Source: CAD feature listing. Evaluate the final solid. Frame: model axes, mm. A direction names the side the tool comes from. Round coordinates to 2 decimals unless told otherwise and drop trailing zeros. Loops run counter-clockwise (first coordinate to the right, second up) from the corner with the lowest first, then second, coordinate; pieces in that order, holes last. Notation, with made-up numbers: (-39, -26.75) - (-26, -26.75) arc R23 ccw to (-26, -5.75) - close; hole circle Ø8 at (85, 48.5). An arc over 180 degrees is marked (long way). Use CSV: the item, a comma, the result in double quotes. Start each with the question number.
from build123d import *

# Parameters (mm, degrees)
F0_W     = 250
F0_H     = 300
F1_DEPTH = 300
F2_W     = 250
F2_H     = 250
F3_DEPTH = 250.001


with BuildPart() as f1:
    # F0 (on Front) → F1 (new body)
    with BuildSketch(Plane.XZ):
        with Locations((-125, 150)):
            Rectangle(F0_W, F0_H)
    extrude(amount=F1_DEPTH)

    # F2 (on face) → F3 (cut, through all)
    with BuildSketch(Plane.YZ):
        with Locations((-150, 150)):
            Rectangle(F2_W, F2_H)
    extrude(amount=-F3_DEPTH, mode=Mode.SUBTRACT)


solid = f1.part
1. Mould query, pull axis Z, two halves, no side actions, for faces 1 (the flat face through (-123, -275, 148)), 2 (the flat face through (-127, -148, 0)), 3 (the flat face through (-127, 0, 152)). Classes: +Z half, -Z half, draft (parallel to the pull), parting line (faces both ways), or undercut.
2. Section query A-A on y = -259. Return the cut outline in (x, z), and give its area (3 significant figures).
3. Section query C-C on z = 34. Return the cut outline in (x, y).
4. Line query: line 1 along Z through (x, y) = (-41.5, -211); line 2 along Y through (x, z) = (-95.5, 34.5). Output: solid intervals per line, ascending.
5. Section query B-B on x = -233.5. Return the cut outline in (y, z).
6. Reachability of faces 4 (the flat face through (-123, -152, 275)), 5 (the flat face through (-127, -148, 300)) from +Z, -Z, +X, -X, +Y, -Y: full face, straight path, thin tool, end or side. Return the list, or none.
Values:
1,face 1,"undercut"
1,face 2,"-Z half"
1,face 3,"draft"
2,outline,"(-250, 0) - (0, 0) - (0, 25) - (-250, 25) - close; (-250, 275) - (0, 275) - (0, 300) - (-250, 300) - close"
2,area,"12,500 mm^2"
3,outline,"(-250, -300) - (0, -300) - (0, -275) - (-250, -275) - close; (-250, -25) - (0, -25) - (0, 0) - (-250, 0) - close"
4,line 1,"z = 0 to 25, 275 to 300"
4,line 2,"y = -300 to -275, -25 to 0"
5,outline,"(-300, 0) - (0, 0) - (0, 300) - (-300, 300) - close; hole (-275, 25) - (-25, 25) - (-25, 275) - (-275, 275) - close"
6,face 4,"+X, -X"
6,face 5,"+Z, +X, -X, +Y, -Y"
